Work out the finished part from the listing and answer in its coordinate system (mm). A direction names the side the tool comes from. Round coordinates to 2 decimals unless told otherwise and drop trailing zeros. Loops run counter-clockwise (first coordinate to the right, second up) from the corner with the lowest first, then second, coordinate; pieces in that order, holes last. Notation, with made-up numbers: M 70.25,52 L 108.25,52 A16 ccw 108.25,81 Z; hole C 75.25,43.5 d9. An arc over 180 degrees is marked long. One line per item, written item: value.
```python
from build123d import *

# Parameters (mm, degrees)
SKETCH1_R           = 5
BOSS_EXTRUDE1_DEPTH = 3


with BuildPart() as part:
    # Sketch1 → Boss-Extrude1 (new body)
    with BuildSketch(Plane(origin=(0, 0, 0), x_dir=(0, 0, -1), z_dir=(1, 0, 0))):
        Circle(SKETCH1_R)
    extrude(amount=BOSS_EXTRUDE1_DEPTH)

    # Sketch2 → Cut-Revolve1 (revolve, cut)
    with BuildSketch(Plane(origin=(0, 0, 0), x_dir=(1, 0, 0), z_dir=(0, 1, 0))):
        Polygon((3, 2.635374789), (2.09701047, 2.635374789), (2.09701047, 4.136429685), (0.664185342, 4.136429685), (0.664185342, 0), (3.615122808, 0), (3.615122808, 2.635374789), align=None)
    revolve(axis=Axis((3.615122808, 0, 0), (-1, 0, 0)), mode=Mode.SUBTRACT)


solid = part.part
```
1) Find the intervals of material crossed by probe 1 along Y at (x, z) = (2.3, 0); probe 2 along X at (y, z) = (-0.5, 4); probe 3 along Y at (x, z) = (1.25, 0), in increasing order. Write a range as from..to.
Check values:
probe 1: -5..-2.64, 2.64..5
probe 2: 0..0.66, 2.1..3
probe 3: -5..-4.14, 4.14..5
2) Find section B-B (x = 1.1). Give the vertices of the cut face in (y, z), then the cut area to 3 significant figures.
Check values:
outline: C 0,0 d10; hole C 0,0 d8.27
area: 24.8 mm2
3) Find section D-D (z = -4). Give the vertices of the cut face in (x, y).
Check values:
outline: M 0,-3 L 3,-3 L 3,3 L 0,3 Z; hole M 0.66,-1.05 L 2.1,-1.05 L 2.1,1.05 L 0.66,1.05 Z
4) Find section A-A (z = 0). Give the vertices of the cut face in (x, y).
Check values:
outline: M 0,-5 L 3,-5 L 3,-2.64 L 2.1,-2.64 L 2.1,-4.14 L 0.66,-4.14 L 0.66,4.14 L 2.1,4.14 L 2.1,2.64 L 3,2.64 L 3,5 L 0,5 Z
5) For faces 1 (the face through (2.542, 1.604, 2.091)), 2 (the face through (3, -2, -2)), 3 (the face through (2.097, 3, 0)), determine the directions among +Z, -Z, +X, -X, +Y, -Y from which every point of the face is accessible in a straight line to the end or side of a thin tool.
Check values:
face 1: +X
face 2: +Z, -Z, +X, +Y, -Y
face 3: none
6) Each of these flat-tipped pins is pushed along its axis until it touches: pin 1 (2.5 mm diameter, centred on y = 1, z = 0.5, fed in from +X); pin 2 (1 mm diameter, centred on x = 1.5, z = 3.5, fed in from -Y); pin 3 (1 mm diameter, centred on x = 2.5, y = -1, fed in from -Z). Where does it stop, or does it pass through?
Check values:
pin 1: x = 0.66
pin 2: y = -4
pin 3: z = -4.97
7) The mould has two halves that part along Z. Classify faces 4 (the face through (0, 0, 0)), 5 (the face through (0.664, 0, 0)), 6 (the face through (1.48, -4.88, 1.08)): +Z half, -Z half, draft (parallel to the pull), parting line (faces both ways), or undercut.
Check values:
face 4: draft
face 5: undercut
face 6: parting line
